Design review of the part built by this model. Coordinates are the model's own, in mm. Face numbers are marked on the shaded views. A direction names the side the tool comes from. Coordinates: 2 decimals unless noted, no trailing zeros. Write each loop counter-clockwise with the first axis right and the second up, starting at its lowest first coordinate (ties: lowest second). Pieces come first, ordered by that corner, then holes. Notation, with made-up numbers: (-11, 45) - (45, 45) arc R15 cw to (45, 55) - close; hole circle Ø1 at (44, -15.75). An arc over 180 degrees is marked (long way). Use a Markdown table: item, result.
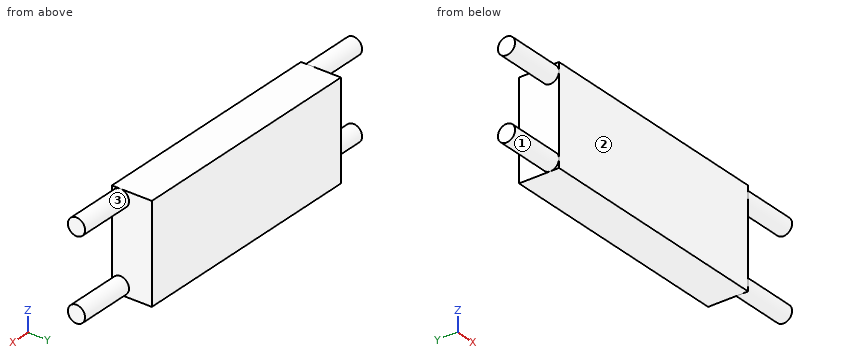
from build123d import *

# Parameters (mm, degrees)
SKETCH1_W           = 43
SKETCH1_H           = 17
BOSS_EXTRUDE1_DEPTH = 7
SKETCH2_R           = 1.5
BOSS_EXTRUDE2_DEPTH = 10


with BuildPart() as part:
    # Sketch1 → Boss-Extrude1 (new body)
    with BuildSketch(Plane(origin=(0, 0, 0), x_dir=(1, 0, 0), z_dir=(0, 1, 0))):
        with Locations((21.5, 8.5)):
            Rectangle(SKETCH1_W, SKETCH1_H)
    extrude(amount=BOSS_EXTRUDE1_DEPTH)

    # Sketch2 → Boss-Extrude2 (add)
    with BuildSketch(Plane(origin=(43, 0, 0), x_dir=(0, 0, -1), z_dir=(1, 0, 0))):
        with Locations((15.5, 1.5)):
            Circle(SKETCH2_R)
        with Locations((1.5, 1.5)):
            Circle(SKETCH2_R)
    boss_extrude2 = extrude(amount=BOSS_EXTRUDE2_DEPTH)

    # Mirror1: Boss-Extrude2 across plane
    add(boss_extrude2.mirror(Plane(origin=(21.5, 0, 0), x_dir=(0, 0, 1), z_dir=(1, 0, 0))))


solid = part.part
(1) Machinability: for the marked faces 1, 2 and 3, which of the approach directions +Z, -Z, +X, -X, +Y, -Y give a long, thin tool a straight path to every point of the face, cutting with its end or side? Answer none if there is none.
Determined:
| item | result |
|---|---|
| face 1 | -X |
| face 2 | +Z, -Z, +X, -X, -Y |
| face 3 | +X |
(2) For pin 1 (1.5 mm diameter, centred on y = 1, z = -4.5, fed in from +X); pin 2 (8 mm diameter, centred on x = -2.5, z = -9, fed in from +Y); pin 3 (4 mm diameter, centred on y = 3, z = -5, fed in from -X), all flat-tipped, find the tip position at first contact; note any pin that passes through.
Determined:
| item | result |
|---|---|
| pin 1 | x = 43 |
| pin 2 | y = 7 |
| pin 3 | x = 0 |
(3) Take a section at A-A on z = -7.5. Write out the cut boundary in (x, y).
Determined:
| item | result |
|---|---|
| outline | (0, 0) - (43, 0) - (43, 7) - (0, 7) - close |
(4) Take a section at B-B on y = 4.25. Write out the cut boundary in (x, z), and give its area (3 significant figures).
Determined:
| item | result |
|---|---|
| outline | (0, -17) - (43, -17) - (43, 0) - (0, 0) - close |
| area | 731 mm2 |
(5) For L1, parallel to X at y = 2.25, z = -4.75; L2, parallel to Z at x = -1, y = 2.75, list the stretches that pass through material, from the lowest coordinate up. Write a range as from..to.
Determined:
| item | result |
|---|---|
| L1 | 0..43 |
| L2 | -16.33..-14.67, -2.33..-0.67 |
